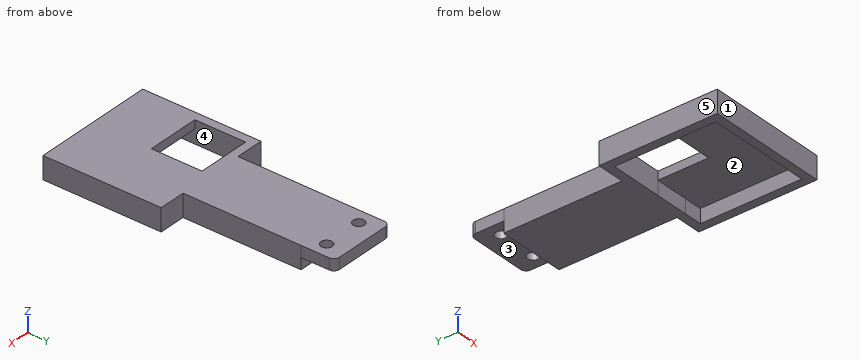
```python
from build123d import *

# Parameters (mm, degrees)
SKETCH_1_R      = 2
EXTRUDE_1_DEPTH = 4
SKETCH_2_W      = 24.000018158
SKETCH_2_H      = 8
EXTRUDE_2_DEPTH = 45
EXTRUDE_START   = -3
EXTRUDE_3_DEPTH = 5
SKETCH_4_W      = 43.5
SKETCH_4_H      = 42
SKETCH_4_W_2    = 19
SKETCH_4_H_2    = 18
EXTRUDE_4_DEPTH = 3


with BuildPart() as part:
    # 草图1 → 凸台-拉伸1 (new body)
    with BuildSketch(Plane.XY):
        with BuildLine():
            Line((49.58322575, -24.029522484), (49.58322575, -14))
            ThreePointArc((49.58322575, -14), (48.997439312, -12.585786438), (47.58322575, -12))
            Line((47.58322575, -12), (27.58322575, -12))
            ThreePointArc((27.58322575, -12), (26.169012187, -12.585786438), (25.58322575, -14))
            Line((25.58322575, -14), (25.58322575, -24))
            Line((25.58322575, -24), (49.58322575, -24.029522484))
        make_face()
        with Locations((30.58322575, -19)):
            Circle(SKETCH_1_R, mode=Mode.SUBTRACT)
        with Locations((44.58322575, -19)):
            Circle(SKETCH_1_R, mode=Mode.SUBTRACT)
    extrude(amount=EXTRUDE_1_DEPTH)

    # 草图2 → 凸台-拉伸2 (add)
    with BuildSketch(Plane(origin=(-0.029483728, -23.968493717, 0), x_dir=(0.9999992434235635, -0.0012301025569531234, 0), z_dir=(-0.0012301025569531234, -0.9999992434235636, 0))):
        with Locations((37.612737934, 0)):
            Rectangle(SKETCH_2_W, SKETCH_2_H)
    extrude(amount=EXTRUDE_2_DEPTH)

    # 草图3 → 凸台-拉伸3 (add)
    with BuildSketch(Plane.XY.offset(4).offset(EXTRUDE_START)):
        Polygon((37.527871134, -66.014727196), (15.527871134, -66.014727196), (15.527871134, -108.014727196), (37.027871134, -108.014727196), (59.027871134, -108.014727196), (59.027871134, -66.014727196), align=None)
        Polygon((37.527871134, -69.014727196), (18.527871134, -69.014727196), (18.527871134, -105.014727196), (37.027871134, -105.014727196), (56.027871134, -105.014727196), (56.027871134, -69.014727196), align=None, mode=Mode.SUBTRACT)
    extrude(amount=-EXTRUDE_3_DEPTH)

    # 草图4 → 凸台-拉伸4 (add)
    with BuildSketch(Plane.XY.offset(1)):
        with Locations((37.277871134, -87.014727196)):
            Rectangle(SKETCH_4_W, SKETCH_4_H)
        with Locations((28.027871134, -78.014727196)):
            Rectangle(SKETCH_4_W_2, SKETCH_4_H_2, mode=Mode.SUBTRACT)
    extrude(amount=EXTRUDE_4_DEPTH)


solid = part.part
```
Source: CAD feature listing. Evaluate the final solid. Frame: model axes, mm. Face numbers are marked on the shaded views. A direction names the side the tool comes from. Coordinates: 2 decimals unless noted, no trailing zeros. Loops run counter-clockwise (first coordinate to the right, second up) from the corner with the lowest first, then second, coordinate; pieces in that order, holes last. Notation, with made-up numbers: M 67.25,85.5 L 106.25,85.5 A36 ccw 106.25,122.5 Z; hole C 16.5,-38.75 d2. An arc over 180 degrees is marked long. Use a Markdown table: item, result. Add a question column.
Q1. Section query C-C, the plane x = 54.5. Return loops of the section in (y, z), and give its area (3 significant figures).
Q2. Section query D-D, the plane x = 29.5. Return loops of the section in (y, z).
Q3. Draft query along Y for the marked faces 1, 2 and 3. Return one class per face: pulls with the +Y half, pulls with the -Y half, needs draft (parallel to the pull), parting line crosses it, or undercut.
Q4. Section query A-A, the plane y = -79. Return loops of the section in (x, z).
Q5. Material intervals for L1, parallel to Y at x = 25, z = -3; L2, parallel to Y at x = 31.5, z = -1.25; L3, parallel to X at y = -80.5, z = -1, sorted ascending.
Q6. Access query for the marked faces 4 and 5. Directions: +Z, -Z, +X, -X, +Y, -Y. A direction counts if a zero-diameter tool reaches every point of the face in a straight line with its end or side. Return the directions, or none.
Q7. Section query B-B, the plane y = -19. Return loops of the section in (x, z), and give its area (3 significant figures).
Q8. First-contact query: pin 1 (1.2 mm diameter, centred on y = -20.5, z = 3, fed in from +X); pin 2 (4.5 mm diameter, centred on y = -17.5, z = 1.5, fed in from -X); pin 3 (2.5 mm diameter, centred on x = 35, z = -1.5, fed in from +Y). Flat tips, straight axial feed; report the tip coordinate or a pass-through.
Result:
| question | item | result |
|---|---|---|
| 1 | outline | M -108.01,-4 L -105.01,-4 L -105.01,1 L -69.01,1 L -69.01,-4 L -66.01,-4 L -66.01,4 L -108.01,4 Z |
| 1 | area | 156 mm2 |
| 2 | outline | M -108.01,-4 L -105.01,-4 L -105.01,1 L -87.01,1 L -87.01,4 L -108.01,4 Z; M -69.01,-4 L -24,-4 L -24,0 L -20.68,0 L -20.68,4 L -69.01,4 Z; M -17.32,0 L -12,0 L -12,4 L -17.32,4 Z |
| 3 | face 1 | pulls with the -Y half |
| 3 | face 2 | undercut |
| 3 | face 3 | needs draft |
| 4 | outline | M 15.53,-4 L 18.53,-4 L 18.53,4 L 15.53,4 Z; M 37.53,1 L 56.03,1 L 56.03,-4 L 59.03,-4 L 59.03,4 L 37.53,4 Z |
| 5 | L1 | y = -108.01 to -105.01, -69.01 to -66.01 |
| 5 | L2 | y = -108.01 to -105.01, -69.01 to -24.01 |
| 5 | L3 | x = 15.53 to 18.53, 56.03 to 59.03 |
| 6 | face 4 | -Z |
| 6 | face 5 | +Z, -Z, -X, +Y, -Y |
| 7 | outline | M 25.58,0 L 28.58,0 L 28.58,4 L 25.58,4 Z; M 32.58,0 L 42.58,0 L 42.58,4 L 32.58,4 Z; M 46.58,0 L 49.58,0 L 49.58,4 L 46.58,4 Z |
| 7 | area | 64.0 mm2 |
| 8 | pin 1 | stops at x = 49.58 |
| 8 | pin 2 | stops at x = 25.58 |
| 8 | pin 3 | stops at y = -24.01 |
